For this review, take the finished solid that the model builds, in its own axes (mm). A direction names the side the tool comes from. Round coordinates to 2 decimals unless told otherwise and drop trailing zeros. Write each loop counter-clockwise with the first axis right and the second up, starting at its lowest first coordinate (ties: lowest second). Pieces come first, ordered by that corner, then holes.
from build123d import *

# Parameters (mm, degrees)
SKETCH1_R           = 1.75
BOSS_EXTRUDE1_DEPTH = 4
FILLET1_R           = 8.25
SKETCH2_W           = 81.75
SKETCH2_H           = 4
BOSS_EXTRUDE2_DEPTH = 24
FILLET3_R           = 8.25
BOSS_EXTRUDE4_DEPTH = 1
BOSS_EXTRUDE6_DEPTH = 22
SKETCH7_R           = 7.5
CUT_EXTRUDE2_DEPTH  = 115
FILLET6_R           = 10


with BuildPart() as part:
    # Sketch1 → Boss-Extrude1 (new body)
    with BuildSketch(Plane(origin=(0, 0, 0), x_dir=(1, 0, 0), z_dir=(0, 1, 0))):
        Polygon((0, 45), (15, 45), (15, 5), (0, 5), (0, 0), (90, 0), (90, 50), (0, 50), align=None)
        with Locations(Location((5.5, 2.5, 0), (0, 0, 270))):
            Circle(SKETCH1_R, mode=Mode.SUBTRACT)
        with Locations(Location((5.5, 47.5, 0), (0, 0, 270))):
            Circle(SKETCH1_R, mode=Mode.SUBTRACT)
        with Locations(Location((81.55, 12, 0), (0, 0, 270))):
            Circle(SKETCH1_R, mode=Mode.SUBTRACT)
        with Locations(Location((81.55, 38, 0), (0, 0, 270))):
            Circle(SKETCH1_R, mode=Mode.SUBTRACT)
    extrude(amount=BOSS_EXTRUDE1_DEPTH)

    # Fillet1
    fillet1_edges = [part.edges().sort_by_distance(p)[0] for p in [
        (90, 2, -50),
        (90, 2, 0),
    ]]
    fillet(fillet1_edges, radius=FILLET1_R)

    # Sketch2 → Boss-Extrude2 (add)
    with BuildSketch(Plane.XY):
        with Locations((40.875, 2)):
            Rectangle(SKETCH2_W, SKETCH2_H)
    extrude(amount=BOSS_EXTRUDE2_DEPTH)

    # Fillet3
    fillet3_edges = [part.edges().sort_by_distance(p)[0] for p in [
        (81.75, 2, 0),
    ]]
    fillet(fillet3_edges, radius=FILLET3_R)

    # Sketch5 → Boss-Extrude4 (add)
    with BuildSketch(Plane(origin=(0, 4, 0), x_dir=(1, 0, 0), z_dir=(0, 1, 0))):
        Polygon((78.896003606, 34.05), (82.418269231, 34.05), (82.418269231, 15), (80.708653846, 15), (80.708653846, 32.096153846), (77.777884615, 32.096153846), align=None)
        Polygon((56.774038462, 34.05), (58.605769231, 34.05), (64.955769231, 19.037439904), (71.305769231, 34.05), (73.1375, 34.05), (65.077884615, 15), (64.833653846, 15), align=None)
        Polygon((31.374038462, 15), (31.374038462, 34.05), (31.732752404, 34.05), (44.318269231, 19.056520433), (44.318269231, 34.05), (46.027884615, 34.05), (46.027884615, 15), (45.638641827, 15), (33.083653846, 29.959134615), (33.083653846, 15), align=None)
        with BuildLine():
            Line((24.779807692, 34.05), (26.489423077, 34.05))
            Line((26.489423077, 34.05), (26.489423077, 21.185907452))
            add(Edge.make_bspline(
                [(26.489423077, 21.185907452), (26.487714463, 20.94802645), (26.484433715, 20.4912659), (26.466393852, 19.833366552), (26.433010208, 19.232634675), (26.384378211, 18.68770427), (26.319498087, 18.200282505), (26.245251919, 17.766603171), (26.155375115, 17.390285757), (26.020030491, 16.967727607), (25.798103714, 16.504302041), (25.464091692, 16.003803293), (25.049167471, 15.566015729), (24.568557562, 15.185817326), (24.018061417, 14.882882968), (23.409015395, 14.66541264), (22.745168684, 14.532765549), (22.284707257, 14.518756151), (22.047475962, 14.511538462)],
                knots=[0, 0, 0, 0, 1.237770943, 2.376671248, 3.424123796, 4.367912054, 5.222547132, 5.982086412, 6.656319012, 7.234008312, 8.288027371, 9.317870876, 10.352700517, 11.413286737, 12.494591526, 13.606319346, 14.766767577, 16, 16, 16, 16], degree=3))
            add(Edge.make_bspline(
                [(22.047475962, 14.511538462), (21.862645469, 14.517420063), (21.490754275, 14.529254234), (20.937266275, 14.625710986), (20.385349806, 14.774388308), (19.832075492, 14.99211672), (19.266512335, 15.28823862), (18.681000534, 15.675687408), (18.068008595, 16.153741858), (17.664239566, 16.518618731), (17.452884615, 16.709615385)],
                knots=[0, 0, 0, 0, 0.848567217, 1.707373443, 2.573483905, 3.470863513, 4.432650262, 5.500696352, 6.691726801, 8, 8, 8, 8], degree=3))
            Line((17.452884615, 16.709615385), (18.460336538, 18.175))
            add(Edge.make_bspline(
                [(18.460336538, 18.175), (18.69276112, 18.014722029), (19.131609036, 17.712096322), (19.776611779, 17.322787254), (20.348096283, 16.989003138), (20.721927753, 16.818901448), (20.895012019, 16.740144231)],
                knots=[0, 0, 0, 0, 1.196737151, 2.259595785, 3.194191475, 4, 4, 4, 4], degree=3))
            add(Edge.make_bspline(
                [(20.895012019, 16.740144231), (20.999973772, 16.698999184), (21.205827143, 16.618304586), (21.520560791, 16.528247625), (21.833498063, 16.47903108), (22.040967226, 16.469879824), (22.142878606, 16.465384615)],
                knots=[0, 0, 0, 0, 1.051806502, 2.062826769, 3.048436908, 4, 4, 4, 4], degree=3))
            add(Edge.make_bspline(
                [(22.142878606, 16.465384615), (22.274502068, 16.470951216), (22.534673123, 16.481954332), (22.912755719, 16.579105387), (23.274477289, 16.72739278), (23.606870712, 16.944515394), (23.913224033, 17.202677841), (24.166005698, 17.514858402), (24.376738129, 17.860838972), (24.503555031, 18.1883436), (24.584353004, 18.487029259), (24.635633573, 18.761529612), (24.680475425, 19.082448517), (24.719563586, 19.450169036), (24.742447919, 19.86542737), (24.768123361, 20.327004205), (24.777404852, 20.83606327), (24.778982306, 21.190997165), (24.779807692, 21.37671274)],
                knots=[0, 0, 0, 0, 0.997221856, 1.971139923, 2.944579524, 3.951425367, 4.971190333, 5.972282193, 6.985401279, 8.033996657, 8.624075553, 9.332086008, 10.151144245, 11.082816738, 12.137127781, 13.306538797, 14.590673636, 16, 16, 16, 16], degree=3))
            Line((24.779807692, 21.37671274), (24.779807692, 34.05))
        make_face()
    extrude(amount=BOSS_EXTRUDE4_DEPTH)

    # Sketch6 → Boss-Extrude6 (add)
    with BuildSketch(Plane(origin=(0, 4, 0), x_dir=(1, 0, 0), z_dir=(0, 1, 0))):
        Polygon((0, -24), (0, -6), (81.75, -6.039419162), (81.75, -24), align=None)
    extrude(amount=BOSS_EXTRUDE6_DEPTH)

    # Sketch7 → Cut-Extrude2 (cut)
    with BuildSketch(Plane.ZY):
        with Locations((15, 13)):
            Circle(SKETCH7_R)
    extrude(amount=-CUT_EXTRUDE2_DEPTH, mode=Mode.SUBTRACT)

    # Fillet6
    fillet6_edges = [part.edges().sort_by_distance(p)[0] for p in [
        (40.875, 26, 24),
        (40.875, 0, 24),
    ]]
    fillet(fillet6_edges, radius=FILLET6_R)


solid = part.part
(1) We need section B-B, the plane y = 11. Give the boundary of the cut face in (x, z), and give its area (3 significant figures).
Geometry check:
outline: (0, 6) - (81.75, 6.04) - (81.75, 7.77) - (0, 7.77) - close; (0, 22.23) - (81.75, 22.23) - (81.75, 24) - (0, 24) - close
area: 288 mm2
(2) For line 1 along X through (y, z) = (1.7, -12); line 2 along Z through (x, y) = (81.55, 1.7); line 3 along Z through (x, y) = (81.55, 2.3), list the stretches that pass through material, from the lowest coordinate up.
Geometry check:
line 1: x = 15 to 79.8, 83.3 to 90
line 2: z = -50 to -39.75, -36.25 to -13.75, -10.25 to 19.58
line 3: z = -50 to -39.75, -36.25 to -13.75, -10.25 to 20.38
(3) We need section A-A, the plane z = -38. Give the boundary of the cut face in (x, y).
Geometry check:
outline: (15, 0) - (79.8, 0) - (79.8, 4) - (15, 4) - close; (83.3, 0) - (90, 0) - (90, 4) - (83.3, 4) - close
(4) We need section D-D, the plane x = 48. Give the boundary of the cut face in (y, z).
Geometry check:
outline: (0, -50) - (4, -50) - (4, 6.02) - (26, 6.02) - (26, 14) arc R10 ccw to (16, 24) - (10, 24) arc R10 ccw to (0, 14) - close; hole circle Ø15 at (13, 15)
(5) For pin 1 Ø1.2 at (x, y) = (9.5, 1.5) entering from +Z; pin 2 Ø0.8 at (x, y) = (80.5, 4.5) entering from -Z; pin 3 Ø3 at (y, z) = (2, -20) entering from -X, all flat-tipped, find the tip position at first contact; note any pin that passes through.
Geometry check:
pin 1: stops at z = 20.13
pin 2: stops at z = -34.05
pin 3: stops at x = 15
(6) Mouldability with a two-part tool opening along Z and no side actions: class faces 5 (the face through (90, 2, -25)), 6 (the face through (69.164, 4.493, -24.658)), 7 (the face through (41.45, 3.01, 21.15)), 8 (the face through (68.086, 4.493, -26.439)) as pulls with the +Z half, pulls with the -Z half, needs draft (parallel to the pull), parting line crosses it, or undercut.
Geometry check:
face 5: needs draft
face 6: undercut
face 7: pulls with the +Z half
face 8: pulls with the -Z half
(7) We need section C-C, the plane x = 29. Give the boundary of the cut face in (y, z), and give its area (3 significant figures).
Geometry check:
outline: (0, -50) - (4, -50) - (4, 6.01) - (26, 6.01) - (26, 14) arc R10 ccw to (16, 24) - (10, 24) arc R10 ccw to (0, 14) - close; hole circle Ø15 at (13, 15)
area: 472 mm2
(8) For faces 1 (the face through (60.86, 4.49, -24.39)), 2 (the face through (7, 2, -45)), 3 (the face through (81, 5, -27)), 4 (the face through (37.9, 4.5, -26.7)), list the 3-axis set-ups (+Z, -Z, +X, -X, +Y, -Y) from which the entire face can be reached by the end or side of a thin tool; tool diameter is ignored.
Geometry check:
face 1: +Y
face 2: -X, +Y, -Y
face 3: -Z, +X, -X, +Y
face 4: -Z, +Y
